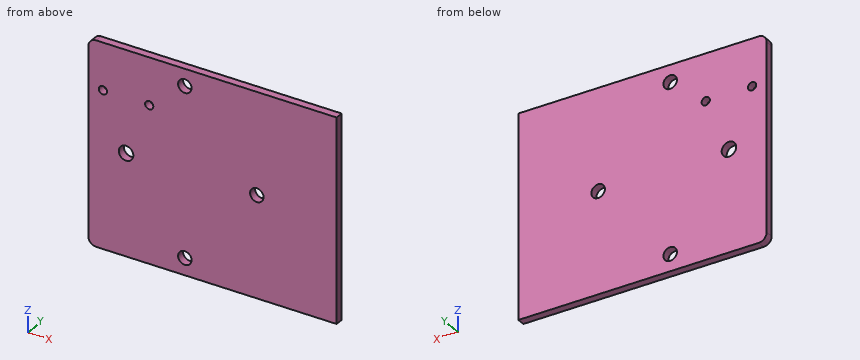
Autodesk Inventor part; units mm, degrees
ref_plane "YZ Plane" through (0, 0, 0) normal (1, 0, 0) x (0, 1, 0)
ref_plane "XZ Plane" through (0, 0, 0) normal (0, 1, 0) x (-1, 0, 0)
ref_plane "XY Plane" through (0, 0, 0) normal (0, 0, 1) x (1, 0, 0)
sketch "Sketch1" plane through (4, 0, 0) normal (0, 1, 0) x (-1, 0, 0)
  circle A0 centre (0, 0) radius 30.16 construction
  line L0 (0, 0) -> (38.16, 0) construction
  line L1 (38.16, 38.16) -> (38.16, -38.16) construction
  line L2 (38.16, 38.16) -> (-30.16, 38.16)
  line L3 (38.16, -38.16) -> (-30.16, -38.16)
  circle A1 centre (27.211, 31.78) radius 2.55
  circle A2 centre (27.211, -31.78) radius 2.55
  circle A3 centre (0, 0) radius 2.55
  line L4 (-30.16, 38.16) -> (-30.16, -38.16)
  line L5 (38.16, 0) -> (49.41, 0) construction
  circle A4 centre (49.41, 0) radius 2.75
  line L6 (40.66, 20.5) -> (58.16, 20.5) construction
  circle A5 centre (58.16, 20.5) radius 1.55
  circle A6 centre (40.66, 20.5) radius 1.55
  line L7 (49.41, 0) -> (63.66, 0) construction
  line L8 (38.16, -38.16) -> (63.66, -38.16)
  line L9 (63.66, -38.16) -> (63.66, 38.16)
  line L10 (63.66, 38.16) -> (38.16, 38.16)
  dimension "d6" = 60.32
  dimension "d4" = 38.16
  dimension "d5" = 76.32
  dimension "d1" = 5.1
  dimension "d3" = 6.38
  dimension "d2" = 10.949
  dimension "d0" = 5.1
  dimension "d10" = 11.25
  dimension "d11" = 5.5
  dimension "d12" = 17.66
  dimension "d13" = 2.5
  dimension "d14" = 17.5
  dimension "d15" = 3.1
  dimension "d16" = 3.1
  dimension "d17" = 14.25
extrude "Extrusion1" add sketch "Sketch1" along normal blind 3
fillet "Fillet1" radius 3 2 edges at (-59.66, 1.5, 38.16) (-59.66, 1.5, -38.16)
properties part number "Tapa B1" material "Polycarbonate, Clear"
The model under review builds one solid part; all positions refer to its coordinate system, in mm. Coordinates: 2 decimals unless noted, no trailing zeros. Write each loop counter-clockwise with the first axis right and the second up, starting at its lowest first coordinate (ties: lowest second). Pieces come first, ordered by that corner, then holes. Notation, with made-up numbers: (62, 17.5) - (79, 17.5) arc R11 ccw to (79, 32.5) - close; hole circle Ø11 at (-29, -11.75). An arc over 180 degrees is marked (long way). Answer as a JSON object with one key per item and string values. Group by question number.
1. Add section A-A (x = 4). Give the boundary of the cut face in (y, z), plus the area to 3 significant figures.
2. Clearance check with a flat-ended pin moving along its axis: pin 1 Ø5 at (x, z) = (-45.41, 0) entering from -Y. State where the tip first meets the part, or that it passes through.
3. To check wall thickness, follow probe 1 along Z at (x, y) = (-45.41, 1.4); probe 2 along Z at (x, y) = (-54, 0.6); probe 3 along Z at (x, y) = (-21, 2.75). State the ranges of each line that lie inside material, in increasing order.
4. Add section B-B (z = 31.78). Give the boundary of the cut face in (x, y), plus the area to 3 significant figures.
5. Add section C-C (z = 0). Give the boundary of the cut face in (x, y), plus the area to 3 significant figures.
Findings:
{
 "1": {"outline": "(0, -38.16) - (3, -38.16) - (3, -2.55) - (0, -2.55) - close; (0, 2.55) - (3, 2.55) - (3, 38.16) - (0, 38.16) - close", "area": "214 mm²"},
 "2": {"pin 1": "through"},
 "3": {"probe 1": "-38.16 to -2.75, 2.75 to 38.16", "probe 2": "-38.16 to 18.96, 22.04 to 38.16", "probe 3": "-38.16 to -33.05, -30.51 to 30.51, 33.05 to 38.16"},
 "4": {"outline": "(-59.66, 0) - (-25.76, 0) - (-25.76, 3) - (-59.66, 3) - close; (-20.66, 0) - (34.16, 0) - (34.16, 3) - (-20.66, 3) - close", "area": "266 mm²"},
 "5": {"outline": "(-59.66, 0) - (-48.16, 0) - (-48.16, 3) - (-59.66, 3) - close; (-42.66, 0) - (1.45, 0) - (1.45, 3) - (-42.66, 3) - close; (6.55, 0) - (34.16, 0) - (34.16, 3) - (6.55, 3) - close", "area": "250 mm²"}
}
